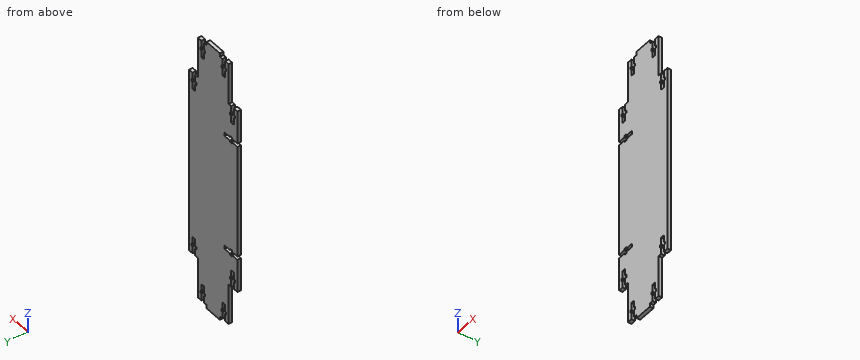
```python
from build123d import *

# Parameters (mm, degrees)
SKETCH_1_W           = 55
SKETCH_1_H           = 160
EXTRUDE_1_DEPTH      = 3
EXTRUDE_2_DEPTH      = 35
EXTRUDE_2_DEPTH_BACK = 195
SKETCH_2_W           = 35
SKETCH_2_H           = 3
EXTRUDE_3_DEPTH      = 3
EXTRUDE_3_DEPTH_BACK = 233
SKETCH_3_W           = 15
SKETCH_3_H           = 3
CUT_EXTRUDE_1_DEPTH  = 3
CUT_EXTRUDE_2_DEPTH  = 3


with BuildPart() as part:
    # Эскиз1 → Бобышка-Вытянуть1 (new body)
    with BuildSketch(Plane(origin=(0, 0, 0), x_dir=(1, 0, 0), z_dir=(0, 1, 0))):
        Rectangle(SKETCH_1_W, SKETCH_1_H)
    extrude(amount=EXTRUDE_1_DEPTH)

    # Эскиз2 → Бобышка-Вытянуть2 (add, two sides: drawn at the far end of the back side and taken through both)
    with BuildSketch(Plane(origin=(0, 0, -80), x_dir=(-1, 0, 0), z_dir=(0, 0, -1)).offset(-EXTRUDE_2_DEPTH_BACK)):
        with Locations((0, 1.5)):
            Rectangle(SKETCH_2_W, SKETCH_2_H)
    extrude(amount=EXTRUDE_2_DEPTH + EXTRUDE_2_DEPTH_BACK)

    # Эскиз3 → Бобышка-Вытянуть3 (add, two sides: drawn at the far end of the back side and taken through both)
    with BuildSketch(Plane(origin=(0, 0, -115), x_dir=(-1, 0, 0), z_dir=(0, 0, -1)).offset(-EXTRUDE_3_DEPTH_BACK)):
        with Locations((0, 1.5)):
            Rectangle(SKETCH_3_W, SKETCH_3_H)
    extrude(amount=EXTRUDE_3_DEPTH + EXTRUDE_3_DEPTH_BACK)

    # Эскиз4 → Вырез-Вытянуть1 (cut)
    with BuildSketch(Plane(origin=(0, 3, 0), x_dir=(1, 0, 0), z_dir=(0, 1, 0))):
        Polygon((-23.5, 80), (-23.5, 74), (-24.75, 74), (-24.75, 71.5), (-23.5, 71.5), (-23.5, 65.5), (-20.5, 65.5), (-20.5, 71.5), (-19.25, 71.5), (-19.25, 74), (-20.5, 74), (-20.5, 80), align=None)
        Polygon((-13.5, 115), (-13.5, 109), (-14.75, 109), (-14.75, 106.5), (-13.5, 106.5), (-13.5, 100.5), (-10.5, 100.5), (-10.5, 106.5), (-9.25, 106.5), (-9.25, 109), (-10.5, 109), (-10.5, 115), align=None)
        Polygon((10.5, 115), (13.5, 115), (13.5, 109), (14.75, 109), (14.75, 106.5), (13.5, 106.5), (13.5, 100.5), (10.5, 100.5), (10.5, 106.5), (9.25, 106.5), (9.25, 109), (10.5, 109), align=None)
        Polygon((20.5, 80), (23.5, 80), (23.5, 74), (24.75, 74), (24.75, 71.5), (23.5, 71.5), (23.5, 65.5), (20.5, 65.5), (20.5, 71.5), (19.25, 71.5), (19.25, 74), (20.5, 74), align=None)
        Polygon((-10.5, -115), (-13.5, -115), (-13.5, -109), (-14.75, -109), (-14.75, -106.5), (-13.5, -106.5), (-13.5, -100.5), (-10.5, -100.5), (-10.5, -106.5), (-9.25, -106.5), (-9.25, -109), (-10.5, -109), align=None)
        Polygon((13.5, -115), (13.5, -109), (14.75, -109), (14.75, -106.5), (13.5, -106.5), (13.5, -100.5), (10.5, -100.5), (10.5, -106.5), (9.25, -106.5), (9.25, -109), (10.5, -109), (10.5, -115), align=None)
        Polygon((-20.5, -80), (-23.5, -80), (-23.5, -74), (-24.75, -74), (-24.75, -71.5), (-23.5, -71.5), (-23.5, -65.5), (-20.5, -65.5), (-20.5, -71.5), (-19.25, -71.5), (-19.25, -74), (-20.5, -74), align=None)
        Polygon((23.5, -80), (23.5, -74), (24.75, -74), (24.75, -71.5), (23.5, -71.5), (23.5, -65.5), (20.5, -65.5), (20.5, -71.5), (19.25, -71.5), (19.25, -74), (20.5, -74), (20.5, -80), align=None)
    extrude(amount=-CUT_EXTRUDE_1_DEPTH, mode=Mode.SUBTRACT)

    # Эскиз5 → Вырез-Вытянуть2 (cut)
    with BuildSketch(Plane(origin=(0, 3, 0), x_dir=(1, 0, 0), z_dir=(0, 1, 0))):
        Polygon((-27.5, 51.5), (-21.5, 51.5), (-21.5, 52.75), (-19, 52.75), (-19, 51.5), (-13, 51.5), (-13, 48.5), (-19, 48.5), (-19, 47.25), (-21.5, 47.25), (-21.5, 48.5), (-27.5, 48.5), align=None)
        Polygon((-27.5, -48.5), (-27.5, -51.5), (-21.5, -51.5), (-21.5, -52.75), (-19, -52.75), (-19, -51.5), (-13, -51.5), (-13, -48.5), (-19, -48.5), (-19, -47.25), (-21.5, -47.25), (-21.5, -48.5), align=None)
    extrude(amount=-CUT_EXTRUDE_2_DEPTH, mode=Mode.SUBTRACT)


solid = part.part
```
Here's how the part is built. I have some questions about the finished solid (model axes, mm). Coordinates: 2 decimals unless noted, no trailing zeros. Write each loop counter-clockwise with the first axis right and the second up, starting at its lowest first coordinate (ties: lowest second). Pieces come first, ordered by that corner, then holes. Notation, with made-up numbers: (56, 46.25) -> (90, 46.25) arc R27 cw to (90, 77.25) -> close; hole circle Ø3 at (73, 20). An arc over 180 degrees is marked (long way). Use a Markdown table: item, result. Add a question column.
(1) Please list where these lines run through material, in increasing order: line 1 (Z direction, x = 24.5, y = 1.1); line 2 (X direction, y = 2.6, z = -72); line 3 (Z direction, x = -24, y = 0.9).
(2) If we section it at A-A, the plane z = 69.5: Write out the boundary of the cut face in (x, y), and give its area (3 significant figures).
(3) I'm going to push flat-ended pins straight in: P1, Ø1.5, axis at x = 12, y = 0.5, coming from the +Z side; P2, Ø1.4, axis at x = -20, y = 1, coming from the -Z side; P3, Ø1.4, axis at x = -20, y = 2, coming from the +Z side; P4, Ø3, axis at x = 1.5, z = -38.5, coming from the -Y side. Where does each tip first touch, or does it pass through?
Outcome:
| question | item | result |
|---|---|---|
| 1 | line 1 | z = -80 to -74, -71.5 to 71.5, 74 to 80 |
| 1 | line 2 | x = -27.5 to -24.75, -19.25 to 19.25, 24.75 to 27.5 |
| 1 | line 3 | z = -80 to -74, -71.5 to -51.5, -48.5 to 48.5, 51.5 to 71.5, 74 to 80 |
| 2 | outline | (-27.5, 0) -> (-23.5, 0) -> (-23.5, 3) -> (-27.5, 3) -> close; (-20.5, 0) -> (20.5, 0) -> (20.5, 3) -> (-20.5, 3) -> close; (23.5, 0) -> (27.5, 0) -> (27.5, 3) -> (23.5, 3) -> close |
| 2 | area | 147 mm^2 |
| 3 | P1 | stops at z = 100.5 |
| 3 | P2 | stops at z = -80 |
| 3 | P3 | stops at z = 80 |
| 3 | P4 | stops at y = 0 |
